Geometry check sheet. Reference: the model listing, model coordinates, mm. A direction names the side the tool comes from. Round coordinates to 2 decimals unless told otherwise and drop trailing zeros. Loops run counter-clockwise (first coordinate to the right, second up) from the corner with the lowest first, then second, coordinate; pieces in that order, holes last.
Autodesk Fusion 360 part; units mm, degrees
sketch "Sketch1" plane through (0, 0, 0) normal (0, 0, 1) x (1, 0, 0)
  line L0 (6, -11.35) -> (-6, -11.35)
  line L1 (-6, -11.35) -> (-6, 11.35)
  line L2 (-6, 11.35) -> (6, 11.35)
  line L3 (6, 11.35) -> (6, -11.35)
  line L4 (6, -11.35) -> (-6, 11.35) construction
  line L5 (-6, -11.35) -> (6, 11.35) construction
  dimension "d1" = 12
  dimension "d2" = 22.7
extrude "Extrude1" add sketch "Sketch1" along normal blind 16.8 makes body 1
sketch "Sketch2" plane through (0, 0, 16.8) normal (0, 0, 1) x (-1, 0, 0)
  line L0 (-6, -11.35) -> (6, -11.35)
  line L1 (6, -11.35) -> (6, 11.35)
  line L2 (6, 11.35) -> (-6, 11.35)
  line L3 (-6, 11.35) -> (-6, -11.35)
  line L4 (-6, 16.35) -> (6, 16.35)
  line L5 (6, 16.35) -> (6, -16.35)
  line L6 (6, -16.35) -> (-6, -16.35)
  line L7 (-6, -16.35) -> (-6, 16.35)
  line L8 (-6, 16.35) -> (6, -16.35) construction
  line L9 (6, 16.35) -> (-6, -16.35) construction
  dimension "d5" = 12
  dimension "d6" = 32.7
extrude "Extrude2" add sketch "Sketch2" along normal blind 2.5 separate body contours L0 L5 L6 L7 | L2 L4 L5 L7 makes body 2 at (2, -14.6833, 16.8) makes body 3 at (2, 13.0167, 16.8)
extrude "Extrude3" add 1 faces at (2, -3.7833, 16.8) along direction (0, 0, 1) blind 6.6 on bodies 1 bodies 1 2 3
sketch "Sketch3" plane through (0, 0, 23.4) normal (0, 0, 1) x (-1, 0, 0)
  line L0 (-6, -11.35) -> (6, -11.35)
  line L1 (6, -11.35) -> (6, 11.35)
  line L2 (6, 11.35) -> (-6, 11.35)
  line L3 (-6, 11.35) -> (-6, -11.35)
  circle A0 centre (0, -11.35) radius 6
  circle A1 centre (0, -5.35) radius 6
extrude "Extrude4" add sketch "Sketch3" along normal blind 4.4 contours A0 A1 | A0 A1 bodies 1
sketch "Sketch4" plane through (0, 0, 27.8) normal (0, 0, 1) x (-1, 0, 0)
  circle A0 centre (0, -5.35) radius 6
  circle A1 centre (0, -5.35) radius 5
  line L0 (5, -5.35) -> (21, -5.35)
  circle A2 centre (21.6, -5.3517) radius 0.6
  circle A3 centre (21.6, -5.3517) radius 2.75
  line L1 (0, -10.35) -> (21.8829, -8.0871)
  line L2 (0, -0.35) -> (21.8833, -2.6163)
  dimension "d13" = 10
  dimension "d14" = 16
  dimension "d15" = 1.2
  dimension "d16" = 5.5
extrude "Extrude5" add sketch "Sketch4" along normal blind 2 contours A0 A1 L0 L2 | A0 L0 A3 L1 | A0 A1 L0 L1 | A0 L0 A3 L2 | A1 L1 L2 | A3 bodies 1
1) Sectioned sample at D-D, the plane y = -10. Record the cut outline in (x, z), then the cut area to 3 significant figures.
Report:
outline: (-6, 0) - (6, 0) - (6, 23.4) - (-6, 23.4) - close
area: 281 mm2
2) Mould release check, pull along X, two halves, no side actions. Record for faces 1 (the face through (0, -5, 23.4)), 2 (the face through (6, 0, 12)), 3 (the face through (-21, 5.4, 28.8)), 4 (the face through (1.301, -0.507, 25.569)): +X half, -X half, draft (parallel to the pull), parting line (faces both ways), or undercut.
Report:
face 1: draft
face 2: +X half
face 3: undercut
face 4: parting line
3) Access from +Z, -Z, +X, -X, +Y, -Y to the whole of each face (thin tool, end or side, straight path). Record for faces 5 (the face through (0, 11.35, 8)), 6 (the face through (0, 11.35, 21)), 7 (the face through (0, -11.35, 21)), 8 (the face through (5, 5.46, 28.79)), 9 (the face through (-5, 10, 23.4)).
Report:
face 5: -Z, +X, -X, +Y
face 6: +Z, +X, -X, +Y
face 7: +Z, +X, -X, -Y
face 8: +Z, +X
face 9: -X, +Y
4) Sectioned sample at C-C, the plane x = -5. Record the cut outline in (y, z), then the cut area to 3 significant figures.
Report:
outline: (-16.35, 16.8) - (-11.35, 16.8) - (-11.35, 0) - (11.35, 0) - (11.35, 16.8) - (16.35, 16.8) - (16.35, 19.3) - (11.35, 19.3) - (11.35, 23.4) - (8.67, 23.4) - (8.67, 27.8) - (9.83, 27.8) - (9.83, 29.8) - (0.87, 29.8) - (0.87, 27.8) - (2.03, 27.8) - (2.03, 23.4) - (-11.35, 23.4) - (-11.35, 19.3) - (-16.35, 19.3) - close
area: 603 mm2
5) Sectioned sample at A-A, the plane y = 6.5. Record the cut outline in (x, z).
Report:
outline: (-24.1, 27.8) - (-5.89, 27.8) - (-5.89, 23.4) - (-6, 23.4) - (-6, 0) - (6, 0) - (6, 23.4) - (5.89, 23.4) - (5.89, 27.8) - (4.87, 27.8) - (4.87, 29.8) - (-24.1, 29.8) - close
6) Gauge pin test, flat ends, axial feed: pin 1 (2 mm diameter, centred on x = 2, z = 22, fed in from +Y); pin 2 (3.5 mm diameter, centred on x = -1, z = 22, fed in from -Y); pin 3 (10 mm diameter, centred on x = -10, y = 5, fed in from -Z); pin 4 (5 mm diameter, centred on y = -0.5, z = 23.5, fed in from -X). Record the tip position at first contact, or that the pin passes through.
Report:
pin 1: stops at y = 11.35
pin 2: stops at y = -11.35
pin 3: stops at z = 0
pin 4: stops at x = -6
7) Sectioned sample at B-B, the plane z = 12. Record the cut outline in (x, y).
Report:
outline: (-6, -11.35) - (6, -11.35) - (6, 11.35) - (-6, 11.35) - close
8) Scan lines: line 1 along X through (y, z) = (-1.5, 7.75); line 2 along Z through (x, y) = (-2, -9.5); line 3 along Y through (x, z) = (-1.5, 20). Record each from-to range of solid material in increasing order.
Report:
line 1: x = -6 to 6
line 2: z = 0 to 23.4
line 3: y = -11.35 to 11.35
